from build123d import *

# Parameters (mm, degrees)
SKETCH_1_W          = 30
SKETCH_1_H          = 30
EXTRUDE_1_DEPTH     = 4.5
SKETCH_2_R          = 5
SKETCH_2_R_2        = 1.6
CUT_EXTRUDE_1_DEPTH = 22.685248442
CUT_EXTRUDE_2_DEPTH = 2.5
CUT_EXTRUDE_3_DEPTH = 8
CUT_EXTRUDE_4_DEPTH = 9.45
CUT_EXTRUDE_5_DEPTH = 2.5
FILLET_1_R          = 0.2
FILLET_2_R          = 0.2
CHAMFER_1_SIZE      = 0.5
FILLET_3_R          = 0.5


with BuildPart() as part:
    # 草图1 → 凸台-拉伸1 (new body)
    with BuildSketch(Plane(origin=(0, 0, 0), x_dir=(0, 0, -1), z_dir=(1, 0, 0))):
        Rectangle(SKETCH_1_W, SKETCH_1_H)
    extrude(amount=EXTRUDE_1_DEPTH)

    # 草图2 → 切除-拉伸1 (cut, through all)
    with BuildSketch(Plane(origin=(4.5, 0, 0), x_dir=(0, 0, -1), z_dir=(1, 0, 0))):
        with Locations((-7.5, 0)):
            Circle(SKETCH_2_R)
        with Locations((10.3, 0)):
            Circle(SKETCH_2_R_2)
    extrude(amount=-CUT_EXTRUDE_1_DEPTH, mode=Mode.SUBTRACT)

    # 草图3 → 切除-拉伸2 (cut)
    with BuildSketch(Plane(origin=(4.5, 0, 0), x_dir=(0, 0, -1), z_dir=(1, 0, 0))):
        with BuildLine():
            Line((10.3, 3), (15, 3))
            Line((15, 3), (15, -3))
            Line((15, -3), (10.3, -3))
            ThreePointArc((10.3, -3), (7.3, 0), (10.3, 3))
        make_face()
    extrude(amount=-CUT_EXTRUDE_2_DEPTH, mode=Mode.SUBTRACT)

    # 草图4 → 切除-拉伸3 (cut)
    with BuildSketch(Plane.XZ.offset(15)):
        with BuildLine():
            Line((1.7, 5.55), (1.7, 9.45))
            Line((1.7, 9.45), (2.944409721, 9.45))
            ThreePointArc((2.944409721, 9.45), (3.411838473, 9.280042303), (3.822875656, 9))
            Line((3.822875656, 9), (4.5, 9))
            Line((4.5, 9), (4.5, 6))
            Line((4.5, 6), (3.822875656, 6))
            ThreePointArc((3.822875656, 6), (3.411838473, 5.719957697), (2.944409721, 5.55))
            Line((2.944409721, 5.55), (1.7, 5.55))
        make_face()
    cut_extrude_3 = extrude(amount=-CUT_EXTRUDE_3_DEPTH, mode=Mode.SUBTRACT)

    # 镜向1: 切除-拉伸3 across plane
    add(cut_extrude_3.mirror(Plane.ZX), mode=Mode.SUBTRACT)

    # 草图5 → 切除-拉伸4 (cut)
    with BuildSketch(Plane.XZ.offset(15)):
        with BuildLine():
            Line((1.7, -9.45), (1.7, -5.55))
            Line((1.7, -5.55), (2.944409721, -5.55))
            ThreePointArc((2.944409721, -5.55), (3.411838473, -5.719957697), (3.822875656, -6))
            Line((3.822875656, -6), (4.5, -6))
            Line((4.5, -6), (4.5, -9))
            Line((4.5, -9), (3.822875656, -9))
            ThreePointArc((3.822875656, -9), (3.411838473, -9.280042303), (2.944409721, -9.45))
            Line((2.944409721, -9.45), (1.7, -9.45))
        make_face()
    cut_extrude_4 = extrude(amount=-CUT_EXTRUDE_4_DEPTH, mode=Mode.SUBTRACT)

    # 镜向2: 切除-拉伸4 across plane
    add(cut_extrude_4.mirror(Plane.ZX), mode=Mode.SUBTRACT)

    # 草图6 → 切除-拉伸5 (cut)
    with BuildSketch(Plane.ZY):
        with BuildLine():
            Line((-3.5, 13), (3.5, 13))
            Line((3.5, 13), (3.5, 5.744562647))
            ThreePointArc((3.5, 5.744562647), (0.5, 0), (3.5, -5.744562647))
            Line((3.5, -5.744562647), (3.5, -13))
            Line((3.5, -13), (-3.5, -13))
            Line((-3.5, -13), (-3.5, -3.5))
            Line((-3.5, -3.5), (-7, -3.5))
            Line((-7, -3.5), (-7, 3.5))
            Line((-7, 3.5), (-3.5, 3.5))
            Line((-3.5, 3.5), (-3.5, 13))
        make_face()
    extrude(amount=-CUT_EXTRUDE_5_DEPTH, mode=Mode.SUBTRACT)

    # 圆角1
    fillet_1_edges = [part.edges().sort_by_distance(p)[0] for p in [
        (4.5, 0, 15),
        (4.5, 15, 0),
        (4.5, -15, 12),
        (4.5, 9, -15),
        (4.5, 0, -7.3),
        (4.5, -3, -12.65),
        (4.5, 3, -12.65),
        (2, 0, -15),
        (3.25, 3, -15),
        (3.25, -3, -15),
        (4.5, -15, 0),
        (4.5, -9, -15),
        (0, -15, 0),
        (0, 0, 15),
        (0, 15, 0),
        (0, 0, -15),
        (4.5, 15, 12),
        (4.5, 15, -12),
        (2.25, -15, -15),
        (2.25, -15, 15),
        (2.25, 15, 15),
        (2.25, 15, -15),
        (4.5, -15, -12),
    ]]
    fillet(fillet_1_edges, radius=FILLET_1_R)

    # 圆角2
    fillet_2_edges = [part.edges().sort_by_distance(p)[0] for p in [
        (0, 8.25, -3.5),
        (0, 3.5, -5.25),
        (0, 0, -7),
        (0, -3.5, -5.25),
        (0, -8.25, -3.5),
        (0, -13, 0),
        (0, -9.372281323, 3.5),
        (0, 0, 0.5),
        (0, 9.372281323, 3.5),
        (0, 13, 0),
    ]]
    fillet(fillet_2_edges, radius=FILLET_2_R)

    # 倒角1
    chamfer_1_edges = [part.edges().sort_by_distance(p)[0] for p in [
        (0, 0, 12.5),
    ]]
    chamfer(chamfer_1_edges, length=CHAMFER_1_SIZE)

    # 圆角3
    fillet_3_edges = [part.edges().sort_by_distance(p)[0] for p in [
        (4.5, 0, 12.5),
    ]]
    fillet(fillet_3_edges, radius=FILLET_3_R)


solid = part.part
Build history of the part. All positions in model axes, mm. A direction names the side the tool comes from. Coordinates: 2 decimals unless noted, no trailing zeros. Write each loop counter-clockwise with the first axis right and the second up, starting at its lowest first coordinate (ties: lowest second). Pieces come first, ordered by that corner, then holes.
(1) Drill centre lines: line 1 (Z direction, x = 2.7, y = 10); line 2 (Y direction, x = 1.05, z = -10.3); line 3 (Y direction, x = 1.5, z = -5.25). Where is each one in solid material? Low to high.
(2) Cut at B-B on z = 7.5. List the corners of the cut face in (x, y), and give its area (3 significant figures).
(3) Mould opens along X. For faces 1 (the cylindrical face through (2.27, 1.5, 2.73)), 2 (the flat face through (4.5, 0, 0)), 3 (the flat face through (0, 7, -6)), 4 (the flat face through (2, -11, 9.45)) say: pulls with the +X half, pulls with the -X half, needs draft (parallel to the pull), parting line crosses it, or undercut.
(4) Cut at A-A on y = 0. State how many separate pieces and enclosed holes the cut face has, and give its area (3 significant figures).
(5) 3-axis set-ups, long thin cutter, end or side, ignore diameter. For faces 5 (the flat face through (3, -5.55, -7)), 6 (the flat face through (1, 0, -7)), 7 (the flat face through (1.7, 11, 7)), 8 (the flat face through (3, 3, -13)): which of +Z, -Z, +X, -X, +Y, -Y reach the whole face in a straight line?
(6) Pin check, flat tips, straight feed: pin 1 Ø3 at (y, z) = (8, -8) entering from +X; pin 2 Ø1.4 at (x, z) = (3, -7) entering from +Y; pin 3 Ø3 at (y, z) = (0, -10.3) entering from -X. Stop position of each tip, or through.
Working result:
1. line 1: z = -15 to -9.45, -5.55 to 5.55, 9.45 to 15
1. line 2: y = -15 to -1.6, 1.6 to 15
1. line 3: y = -15 to -3.5, 3.5 to 15
2. outline: (0, -14.8) arc R0.2 ccw to (0.2, -15) - (1.7, -15) - (1.7, -7) - (4.5, -7) - (4.5, -5.5) arc R0.5 ccw to (4, -5) - (0.5, -5) - (0, -5.5) - close; (0, 5.5) - (0.5, 5) - (4, 5) arc R0.5 ccw to (4.5, 5.5) - (4.5, 7) - (1.7, 7) - (1.7, 15) - (0.2, 15) arc R0.2 ccw to (0, 14.8) - close
2. area: 44.8 mm2
3. face 1: needs draft
3. face 2: pulls with the +X half
3. face 3: pulls with the -X half
3. face 4: undercut
4. separate pieces: 3
4. enclosed holes: 0
4. area: 45.2 mm2
5. face 5: -Y
5. face 6: -X
5. face 7: +Y
5. face 8: -Z, +X
6. pin 1: stops at x = 4.5
6. pin 2: stops at y = 5.55
6. pin 3: passes through
